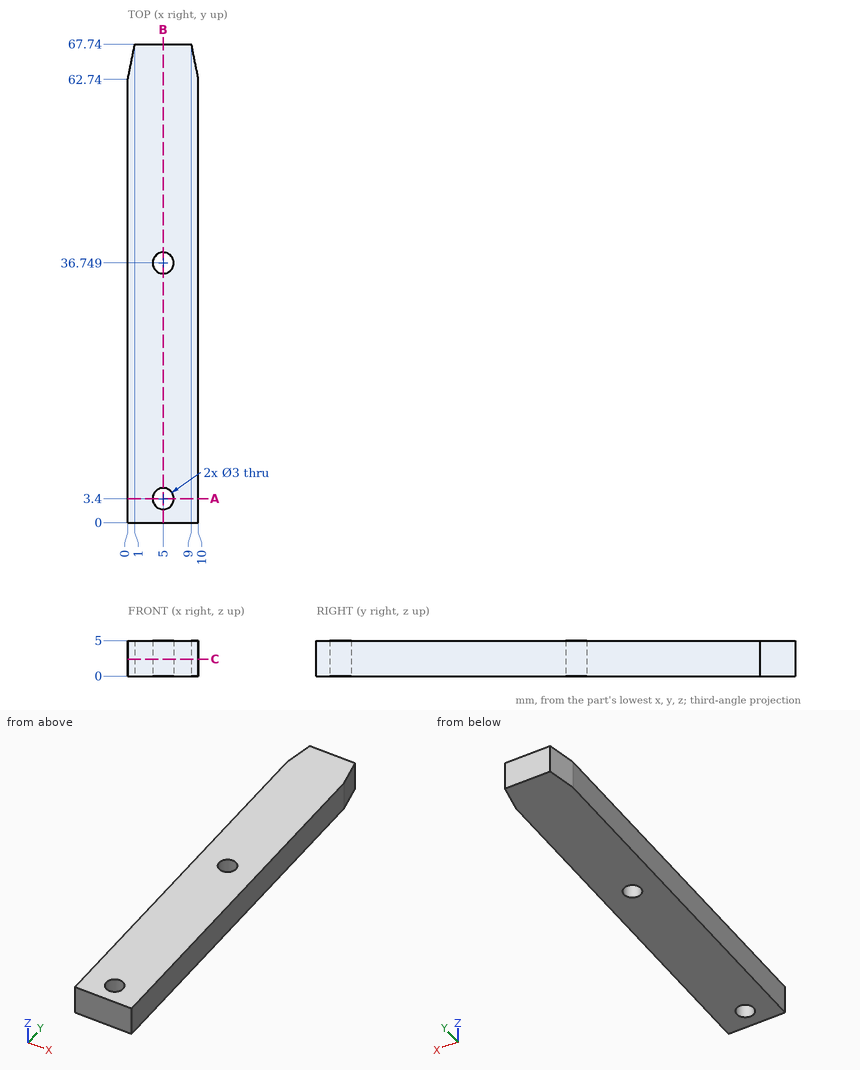
Here's the drawing with two shaded views (mm, measured from the low corner). I have some questions. Coordinates: 2 decimals unless noted, no trailing zeros. Loops run counter-clockwise (first coordinate to the right, second up) from the corner with the lowest first, then second, coordinate; pieces in that order, holes last. Notation, with made-up numbers: M -19,36 L 32,36 A17 ccw 32,55 Z; hole C 64.25,26 d9. An arc over 180 degrees is marked long. Return JSON: item names as keys, results as strings. Group by question number.
Item 1: Imagine slicing it at B-B (x = 5). Please give me the cut outline in (y, z), and give its area (3 significant figures).
Item 2: If I drill on L1, parallel to Y at x = 5, z = 2.8; L2, parallel to X at y = 3.4, z = 1.75; L3, parallel to Y at x = 5.5, z = 2.8 (1 decimal), over which ranges is the centre line in solid material (lowest first)? Write a range as from..to.
Item 3: Imagine slicing it at C-C (z = 2.4). Please give me the cut outline in (x, y), and give its area (3 significant figures).
Item 4: Imagine slicing it at A-A (y = 3.4). Please give me the cut outline in (x, z).
Verdict:
{
 "1": {"outline": "M 0,0 L 1.9,0 L 1.9,5 L 0,5 Z; M 4.9,0 L 35.25,0 L 35.25,5 L 4.9,5 Z; M 38.25,0 L 67.74,0 L 67.74,5 L 38.25,5 Z", "area": "309 mm^2"},
 "2": {"L1": "y = 0..1.9, 4.9..35.25, 38.25..67.74", "L2": "x = 0..3.5, 6.5..10", "L3": "y = 0..2, 4.8..35.3, 38.2..67.7"},
 "3": {"outline": "M 0,0 L 10,0 L 10,62.74 L 9,67.74 L 1,67.74 L 0,62.74 Z; hole C 5,3.4 d3; hole C 5,36.75 d3", "area": "658 mm^2"},
 "4": {"outline": "M 0,0 L 3.5,0 L 3.5,5 L 0,5 Z; M 6.5,0 L 10,0 L 10,5 L 6.5,5 Z"}
}
